Can you work these out from the drawing? Everything is in mm from the part's minimum corner. A direction names the side the tool comes from. Give positions to 0.01 mm unless a question says otherwise; leave off trailing zeros. Loops run counter-clockwise (first coordinate to the right, second up) from the corner with the lowest first, then second, coordinate; pieces in that order, holes last. Notation, with made-up numbers: M 72,83 L 105,83 A34 ccw 105,119 Z; hole C 58,24 d2. An arc over 180 degrees is marked long. Use CSV: the item, a comma, the result in double quotes.
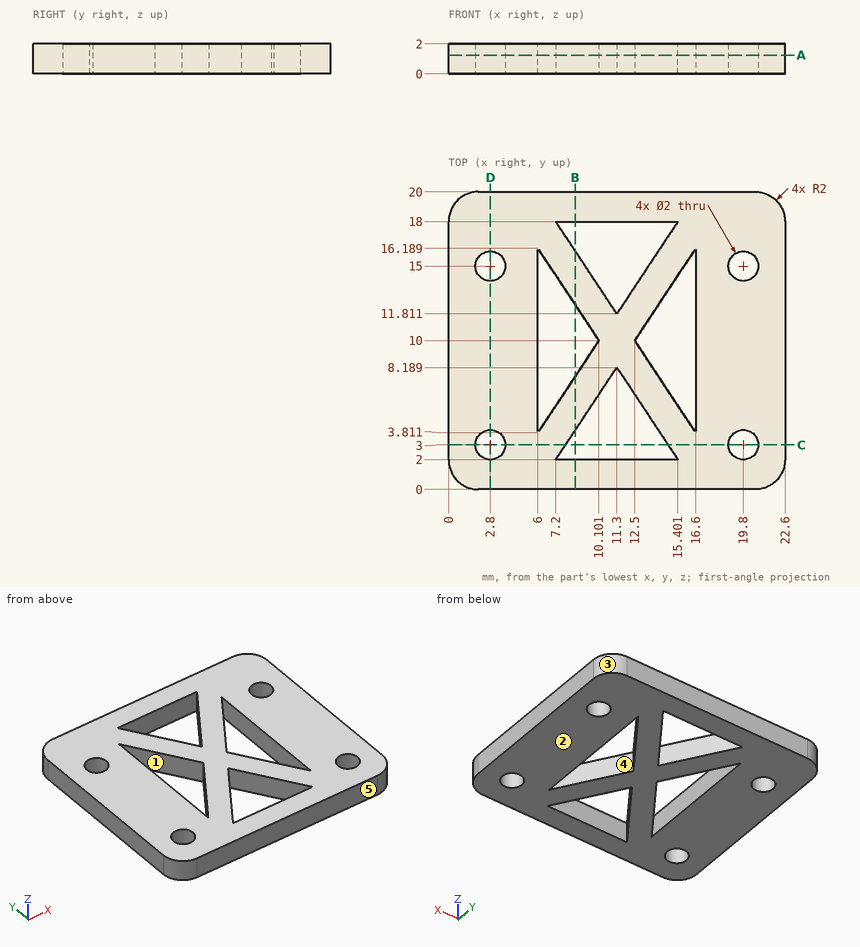
Q1. I want a section at C-C, the plane y = 3. Please give me the cut outline in (x, z).
Model answer:
outline,"M 0,0 L 1.8,0 L 1.8,2 L 0,2 Z; M 3.8,0 L 7.86,0 L 7.86,2 L 3.8,2 Z; M 14.74,0 L 18.8,0 L 18.8,2 L 14.74,2 Z; M 20.8,0 L 22.6,0 L 22.6,2 L 20.8,2 Z"
Q2. I want a section at A-A, the plane z = 1.25. State how many separate pieces and enclosed holes the cut face has.
Model answer:
separate pieces,"1"
enclosed holes,"8"
Q3. I want a section at B-B, the plane x = 8.5. Please give me the cut outline in (y, z) (1 decimal).
Model answer:
outline,"M 0,0 L 2,0 L 2,2 L 0,2 Z; M 4,0 L 7.6,0 L 7.6,2 L 4,2 Z; M 12.4,0 L 16,0 L 16,2 L 12.4,2 Z; M 18,0 L 20,0 L 20,2 L 18,2 Z"
Q4. If we mould it in two halves opening along X, with no side actions, what happens to the marked faces 1, 2 and 3? For each: released by +X, released by -X, zero draft, split by the parting line, or undercut.
Model answer:
face 1,"undercut"
face 2,"zero draft"
face 3,"released by +X"
Q5. I want a section at D-D, the plane x = 2.8. Please give me the cut outline in (y, z), then the cut area to 3 significant figures.
Model answer:
outline,"M 0,0 L 2,0 L 2,2 L 0,2 Z; M 4,0 L 14,0 L 14,2 L 4,2 Z; M 16,0 L 20,0 L 20,2 L 16,2 Z"
area,"32.0 mm2"
Q6. For the marked faces 4 and 5, which set-ups out of +Z, -Z, +X, -X, +Y, -Y let a thin tool reach every point of the face, with its end or its side?
Model answer:
face 4,"+Z, -Z"
face 5,"+Z, -Z, +X, -X, -Y"
Q7. Please list where these lines run through material, in increasing order: L1, parallel to Y at x = 19.8, z = 1.35; L2, parallel to X at y = 3, z = 1.3; L3, parallel to X at y = 8.75, z = 0.4. Write a range as from..to.
Model answer:
L1,"0..2, 4..14, 16..20"
L2,"0..1.8, 3.8..7.86, 14.74..18.8, 20.8..22.6"
L3,"0..6, 9.27..13.33, 16.6..22.6"
